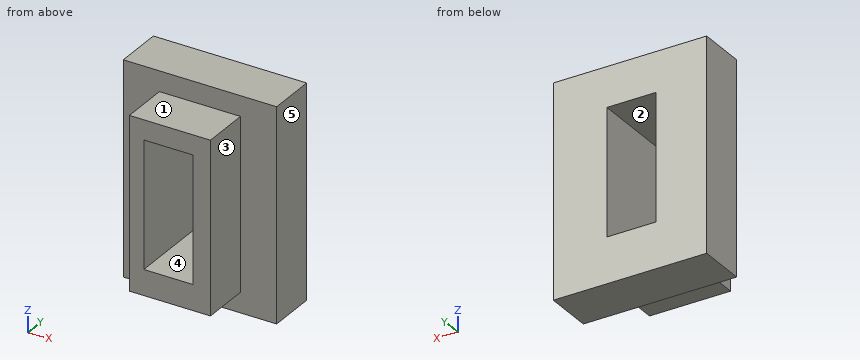
```python
from build123d import *

# Parameters (mm, degrees)
F0_W     = 80.655814
F0_H     = 111.451716
F1_DEPTH = 25.4
F2_W     = 47.660246
F2_H     = 87.988168
F3_DEPTH = 25.4
F4_W     = 42.61583
F4_H     = 90.175256
F4_W_2   = 25.895656
F4_H_2   = 66.464574
F5_DEPTH = 25.4
F6_W     = 25.895656
F6_H     = 66.464574
F7_DEPTH = 31.594573


with BuildPart() as f1:
    # F0 (on Front) → F1 (new body)
    with BuildSketch(Plane.XZ):
        Rectangle(F0_W, F0_H)
    extrude(amount=F1_DEPTH)

    # F2 (on Front) → F3 (join)
    with BuildSketch(Plane.XZ):
        Rectangle(F2_W, F2_H)
    extrude(amount=F3_DEPTH)

    # F4 (on face) → F5 (join)
    with BuildSketch(Plane.XZ.offset(25.4)):
        Rectangle(F4_W, F4_H)
        with Locations((-0.807181, 1.524575)):
            Rectangle(F4_W_2, F4_H_2, mode=Mode.SUBTRACT)
    extrude(amount=F5_DEPTH)

    # F6 (on face) → F7 (cut)
    with BuildSketch(Plane.XZ.offset(25.4)):
        with Locations((-0.807181, 1.524575)):
            Rectangle(F6_W, F6_H)
    extrude(amount=-F7_DEPTH, mode=Mode.SUBTRACT)


solid = f1.part
```
Check sheet for the modelled part. Datum: model origin and axes. Units: mm. Face numbers are marked on the shaded views. A direction names the side the tool comes from. Coordinates: 2 decimals unless noted, no trailing zeros. Loops run counter-clockwise (first coordinate to the right, second up) from the corner with the lowest first, then second, coordinate; pieces in that order, holes last.
1) Release check for a two-part mould opening along Z. For the marked faces 1, 2 and 3 record: released by +Z, released by -Z, zero draft, split by the parting line, or undercut.
2) Sectioned sample at B-B (x = 5.5). Record the boundary of the cut face in (y, z), and give its area (3 significant figures).
3) Gauge pin test, flat ends, axial feed: pin 1 (13 mm diameter, centred on x = 1.5, y = -34, fed in from +Z); pin 2 (8 mm diameter, centred on y = -37.5, z = 8, fed in from +X); pin 3 (7.5 mm diameter, centred on y = -33, z = -5.5, fed in from -X). Record the tip position at first contact, or that the pin passes through.
4) Sectioned sample at C-C (y = -29.5). Record the boundary of the cut face in (x, z) (3 decimals).
5) Sectioned sample at D-D (z = -43). Record the boundary of the cut face in (x, y).
6) Access from +Z, -Z, +X, -X, +Y, -Y to the whole of each face (thin tool, end or side, straight path). Record for the marked faces 4 and 5.
7) Material ranges on probe 1 along Z at (x, y) = (-1, -35); probe 2 along X at (y, z) = (-44.5, 33) (3 decimals); probe 3 along X at (y, z) = (-23, 30) (3 decimals), recorded low to high.
8) Sectioned sample at A-A (z = 6). Record the boundary of the cut face in (x, y) (3 decimals), and give its area (3 significant figures).
Check sheet entries:
1. face 1: released by +Z
1. face 2: undercut
1. face 3: zero draft
2. outline: (-50.8, -45.09) - (-25.4, -45.09) - (-25.4, -55.73) - (0, -55.73) - (0, -31.71) - (-50.8, -31.71) - close; (-50.8, 34.76) - (0, 34.76) - (0, 55.73) - (-25.4, 55.73) - (-25.4, 45.09) - (-50.8, 45.09) - close
2. area: 1,740 mm2
3. pin 1: stops at z = 45.09
3. pin 2: stops at x = 21.31
3. pin 3: stops at x = -21.31
4. outline: (-21.308, -45.088) - (21.308, -45.088) - (21.308, 45.088) - (-21.308, 45.088) - close; hole (-13.755, -31.708) - (12.141, -31.708) - (12.141, 34.757) - (-13.755, 34.757) - close
5. outline: (-40.33, -25.4) - (-21.31, -25.4) - (-21.31, -50.8) - (21.31, -50.8) - (21.31, -25.4) - (40.33, -25.4) - (40.33, 0) - (-40.33, 0) - close
6. face 4: +Y, -Y
6. face 5: +Z, -Z, +X, +Y, -Y
7. probe 1: z = -45.09 to -31.71, 34.76 to 45.09
7. probe 2: x = -21.308 to -13.755, 12.141 to 21.308
7. probe 3: x = -40.328 to -13.755, 12.141 to 40.328
8. outline: (-40.328, -25.4) - (-21.308, -25.4) - (-21.308, -50.8) - (-13.755, -50.8) - (-13.755, 0) - (-40.328, 0) - close; (12.141, -50.8) - (21.308, -50.8) - (21.308, -25.4) - (40.328, -25.4) - (40.328, 0) - (12.141, 0) - close
8. area: 1,820 mm2
